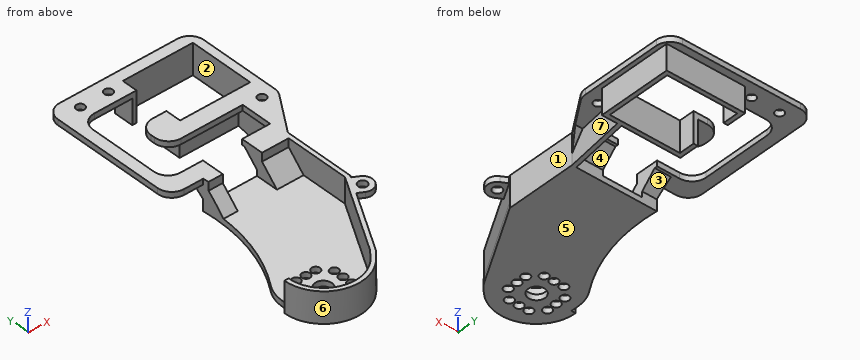
```python
from build123d import *

# Parameters (mm, degrees)
EXTRUDE_1_DEPTH                 = 52
CUT_EXTRUDE_1_REACH             = 124.004
CUT_EXTRUDE_1_DIRECTION_2_DEPTH = 7
SKETCH_3_R                      = 1.5
SKETCH_3_R_2                    = 3
CUT_EXTRUDE_2_DEPTH             = 123.167917229
FILLET_1_R                      = 5
CHAMFER_1_SIZE                  = 5
FILLET_2_R                      = 12.5
EXTRUDE_2_DEPTH                 = 9
EXTRUDE_3_DEPTH                 = 9
EXTRUDE_3_DEPTH_BACK            = 2
CHAMFER_3_SIZE                  = 6
EXTRUDE_START                   = -11
SKETCH_7_R                      = 1.6
EXTRUDE_4_DEPTH                 = 2


with BuildPart() as part:
    # 草图1 → 凸台-拉伸1 (new body)
    with BuildSketch(Plane(origin=(0, 0, 0), x_dir=(0, 0, -1), z_dir=(1, 0, 0))):
        Polygon((0, 0), (0, 58), (-9, 58), (-9, 110), (-7, 110), (-7, 60), (2, 60), (2, 0), align=None)
    extrude(amount=EXTRUDE_1_DEPTH)

    # 草图2 → 切除-拉伸1 (cut, up to next)
    with BuildSketch(Plane(origin=(0, 0, 7), x_dir=(-1, 0, 0), z_dir=(0, 0, -1)), mode=Mode.PRIVATE) as cut_extrude_1_sk1:
        Polygon((-49, 106), (-49, 83), (-24, 83), (-24, 88.5), (-14, 88.5), (-14, 77), (-41, 77), (-41, 66), (-31, 66), (-31, 58), (-17, 58), (-17, 66), (-4, 66), (-4, 100.5), (-24, 100.5), (-24, 106), align=None)
    cut_extrude_1_tool1 = extrude(cut_extrude_1_sk1.sketch, amount=-CUT_EXTRUDE_1_REACH, mode=Mode.PRIVATE) & part.part
    add(cut_extrude_1_tool1.solids().sort_by_distance((25.692202, 84.595066, 7))[0], mode=Mode.SUBTRACT)

    # 草图2 → 切除-拉伸1 direction 2 (cut)
    with BuildSketch(Plane(origin=(0, 0, 7), x_dir=(-1, 0, 0), z_dir=(0, 0, -1))):
        Polygon((-49, 106), (-49, 83), (-24, 83), (-24, 88.5), (-14, 88.5), (-14, 77), (-41, 77), (-41, 66), (-31, 66), (-31, 58), (-17, 58), (-17, 66), (-4, 66), (-4, 100.5), (-24, 100.5), (-24, 106), align=None)
    extrude(amount=CUT_EXTRUDE_1_DIRECTION_2_DEPTH, mode=Mode.SUBTRACT)

    # 草图3 → 切除-拉伸2 (cut, through all)
    with BuildSketch(Plane(origin=(0, 0, -2), x_dir=(-1, 0, 0), z_dir=(0, 0, -1))):
        with Locations(Location((-15.5, 19, 0), (0, 0, 90))):
            Circle(SKETCH_3_R)
        with Locations(Location((-12, 19, 0), (0, 0, 90))):
            Circle(SKETCH_3_R)
        with Locations(Location((-8.5, 19, 0), (0, 0, 90))):
            Circle(SKETCH_3_R)
        with Locations(Location((-8.5, 5, 0), (0, 0, 90))):
            Circle(SKETCH_3_R)
        with Locations(Location((-12, 5, 0), (0, 0, 90))):
            Circle(SKETCH_3_R)
        with Locations(Location((-15.5, 5, 0), (0, 0, 90))):
            Circle(SKETCH_3_R)
        with Locations(Location((-5, 15.5, 0), (0, 0, 90))):
            Circle(SKETCH_3_R)
        with Locations(Location((-5, 12, 0), (0, 0, 90))):
            Circle(SKETCH_3_R)
        with Locations(Location((-5, 8.5, 0), (0, 0, 90))):
            Circle(SKETCH_3_R)
        with Locations(Location((-19, 8.5, 0), (0, 0, 90))):
            Circle(SKETCH_3_R)
        with Locations(Location((-19, 12, 0), (0, 0, 90))):
            Circle(SKETCH_3_R)
        with Locations(Location((-19, 15.5, 0), (0, 0, 90))):
            Circle(SKETCH_3_R)
        with Locations(Location((-8, 105, 0), (0, 0, 90))):
            Circle(SKETCH_3_R)
        with Locations(Location((-47, 76, 0), (0, 0, 90))):
            Circle(SKETCH_3_R)
        with Locations(Location((-18, 105, 0), (0, 0, 90))):
            Circle(SKETCH_3_R)
        with Locations(Location((-12, 12, 0), (0, 0, 90))):
            Circle(SKETCH_3_R_2)
        Polygon((-42, 35), (-22, 0), (-52, 0), (-52, 75), (-42, 60), align=None)
        with BuildLine():
            Line((0, 60), (-11.791303716, 60))
            ThreePointArc((-11.791303716, 60), (-9.662737441, 38.416613409), (0, 19))
            Line((0, 19), (0, 60))
        make_face()
    extrude(amount=-CUT_EXTRUDE_2_DEPTH, mode=Mode.SUBTRACT)

    # 圆角1
    fillet_1_edges = [part.edges().sort_by_distance(p)[0] for p in [
        (0, 60, 8),
        (52, 75, 8),
        (52, 110, 8),
        (14, 88.5, 8),
        (14, 77, 8),
        (4, 66, 8),
        (4, 100.5, 8),
        (0, 110, 8),
    ]]
    fillet(fillet_1_edges, radius=FILLET_1_R)

    # 倒角1
    chamfer_1_edges = [part.edges().sort_by_distance(p)[0] for p in [
        (36.5, 60, 7),
        (14.395651858, 60, 7),
    ]]
    chamfer(chamfer_1_edges, length=CHAMFER_1_SIZE)

    # 圆角2
    fillet_2_edges = [part.edges().sort_by_distance(p)[0] for p in [
        (0, 0, -1),
        (22, 0, -1),
        (0, 19, -1),
    ]]
    fillet(fillet_2_edges, radius=FILLET_2_R)

    # 草图4 → 凸台-拉伸2 (add)
    with BuildSketch(Plane(origin=(0, 0, 7), x_dir=(-1, 0, 0), z_dir=(0, 0, -1))):
        Polygon((-24, 88.5), (-24, 83), (-49, 83), (-49, 106), (-24, 106), (-24, 100.5), (-22.5, 100.5), (-22.5, 107.5), (-50.5, 107.5), (-50.5, 81.5), (-45, 81.5), (-42, 60), (-40.485467906, 60), (-43.485467906, 81.5), (-22.5, 81.5), (-22.5, 88.5), align=None)
    extrude(amount=EXTRUDE_2_DEPTH)

    # 草图6 → 凸台-拉伸3 (add, two sides: drawn at the far end of the back side and taken through both)
    with BuildSketch(Plane.XY.offset(-EXTRUDE_3_DEPTH_BACK)):
        with BuildLine():
            Line((42, 58), (42, 35))
            Line((42, 35), (25.599007583, 6.298263271))
            Line((25.599007583, 6.298263271), (23.114212107, 3.371007649))
            ThreePointArc((23.114212107, 3.371007649), (7.631682503, -0.626289832), (-1.5, 12.5))
            Line((-1.5, 12.5), (0, 12.5))
            ThreePointArc((0, 12.5), (8.295901466, 0.728188095), (22.172088883, 4.581622853))
            Line((22.172088883, 4.581622853), (24.370109829, 7.171038857))
            Line((24.370109829, 7.171038857), (40.5, 35.398346656))
            Line((40.5, 35.398346656), (40.5, 58))
            Line((40.5, 58), (42, 58))
        make_face()
    extrude(amount=EXTRUDE_3_DEPTH + EXTRUDE_3_DEPTH_BACK)

    # 倒角3
    chamfer_3_edges = [part.edges().sort_by_distance(p)[0] for p in [
        (14.462476533, 58, 0),
        (35.75, 58, 0),
    ]]
    chamfer(chamfer_3_edges, length=CHAMFER_3_SIZE)

    # 草图7 → 凸台-拉伸4 (add)
    with BuildSketch(Plane(origin=(0, 0, -2), x_dir=(-1, 0, 0), z_dir=(0, 0, -1)).offset(EXTRUDE_START)):
        with BuildLine():
            Line((-41.58264013, 34.269620228), (-43.736486284, 33.038850997))
            ThreePointArc((-43.736486284, 33.038850997), (-45.038850997, 28.263513716), (-40.263513716, 26.961149003))
            Line((-40.263513716, 26.961149003), (-38.109667562, 28.191918233))
            Line((-38.109667562, 28.191918233), (-41.58264013, 34.269620228))
        make_face()
        with Locations(Location((-42, 30, 0), (0, 0, 90))):
            Circle(SKETCH_7_R, mode=Mode.SUBTRACT)
    extrude(amount=EXTRUDE_4_DEPTH)


solid = part.part
```
For this review, take the finished solid that the model builds, in its own axes (mm). Face numbers are marked on the shaded views. A direction names the side the tool comes from. Coordinates: 2 decimals unless noted, no trailing zeros. Write each loop counter-clockwise with the first axis right and the second up, starting at its lowest first coordinate (ties: lowest second). Pieces come first, ordered by that corner, then holes. Notation, with made-up numbers: (-2, 1) - (49, 1) arc R29 cw to (49, 28) - close; hole circle Ø7 at (48, -7). An arc over 180 degrees is marked (long way). Put each result on its own line as item: value.
1. Add section A-A, the plane x = 29.5. Give the boundary of the cut face in (y, z) (3 decimals), then the cut area to 3 significant figures.
Values found:
outline: (13.125, -2) - (60, -2) - (60, 0) - (16.148, 0) - (16.148, 9) - (13.125, 9) - close; (77, 7) - (81.5, 7) - (81.5, -2) - (83, -2) - (83, 9) - (77, 9) - close; (106, -2) - (107.5, -2) - (107.5, 7) - (110, 7) - (110, 9) - (106, 9) - close
area: 168 mm²
2. For pin 1 (12 mm diameter, centred on x = 35, y = 74.5, fed in from -Z); pin 2 (1 mm diameter, centred on x = 9, z = 8, fed in from -Y); pin 3 (1 mm diameter, centred on x = 31, z = 0, fed in from +Y), all flat-tipped, find the tip position at first contact; note any pin that passes through.
Values found:
pin 1: z = 7
pin 2: y = -1.17
pin 3: y = 107.5
3. Wall thickness on probe 1 along X at (y, z) = (105, 8.35); probe 2 along Y at (x, z) = (28, 5.25); probe 3 along Y at (x, z) = (26, -1): over which ranges is each line inside the solid? List them lowest first.
Values found:
probe 1: 0 to 6.5, 9.5 to 16.5, 19.5 to 24, 49 to 52
probe 2: 10.5 to 13.52, 81.5 to 83, 106 to 107.5
probe 3: 7 to 60, 81.5 to 83, 106 to 107.5
4. Add section C-C, the plane y = 67. Give the boundary of the cut face in (x, z).
Values found:
outline: (0, 7) - (6, 7) - (6, 9) - (0, 9) - close; (41, 7) - (41.46, 7) - (41.46, -2) - (42.98, -2) - (42.98, 7) - (46.67, 7) - (46.67, 9) - (41, 9) - close
5. Add section D-D, the plane y = 30. Give the boundary of the cut face in (x, z), then the cut area to 3 significant figures.
Values found:
outline: (6.54, -2) - (39.14, -2) - (39.14, 7) - (40.4, 7) - (40.4, 9) - (37.42, 9) - (37.42, 0) - (6.54, 0) - close; (43.6, 7) - (45.5, 7) - (45.5, 9) - (43.6, 9) - close
area: 87.1 mm²
6. Machinability: for the marked faces 1, 2, 3 and 4, which of the approach directions +Z, -Z, +X, -X, +Y, -Y give a long, thin tool a straight path to every point of the face, cutting with its end or side? Answer none if there is none.
Values found:
face 1: +Z, -Z, +X
face 2: +Z, -Z
face 3: -Z, -X, +Y
face 4: -Z, -X
7. Mouldability with a two-part tool opening along Y and no side actions: class the marked faces 5, 6 and 7 as released by +Y, released by -Y, zero draft, split by the parting line, or undercut.
Values found:
face 5: zero draft
face 6: released by -Y
face 7: undercut
